```python
from build123d import *

# Parameters (mm, degrees)
SKETCH1_R           = 2.25
SKETCH1_R_2         = 1
SKETCH1_R_3         = 1.65
SKETCH1_W           = 40.6
SKETCH1_H           = 20.8
SKETCH1_W_2         = 23
SKETCH1_H_2         = 12.9
BOSS_EXTRUDE1_DEPTH = 3.175


with BuildPart() as part:
    # Sketch1 → Boss-Extrude1 (new body)
    with BuildSketch(Plane(origin=(0, 0, 0), x_dir=(1, 0, 0), z_dir=(0, 1, 0))):
        with BuildLine():
            Line((-162.38735588, 17.244652891), (-102.38735588, 17.244652891))
            Line((-102.38735588, 17.244652891), (7.61264412, 12.244652891))
            ThreePointArc((7.61264412, 12.244652891), (17.61264412, 2.244652891), (7.61264412, -7.755347109))
            Line((7.61264412, -7.755347109), (-102.38735588, -12.755347109))
            Line((-102.38735588, -12.755347109), (-162.38735588, -12.755347109))
            ThreePointArc((-162.38735588, -12.755347109), (-177.38735588, 2.244652891), (-162.38735588, 17.244652891))
        make_face()
        with Locations(Location((-168.38735588, 7.244652891, 0), (0, 0, 270))):
            Circle(SKETCH1_R, mode=Mode.SUBTRACT)
        with Locations(Location((-168.38735588, -2.755347109, 0), (0, 0, 270))):
            Circle(SKETCH1_R, mode=Mode.SUBTRACT)
        with Locations(Location((-118.78735588, 7.244652891, 0), (0, 0, 270))):
            Circle(SKETCH1_R, mode=Mode.SUBTRACT)
        with Locations(Location((-118.78735588, -2.755347109, 0), (0, 0, 270))):
            Circle(SKETCH1_R, mode=Mode.SUBTRACT)
        with Locations(Location((-15.58735588, 2.244652891, 0), (0, 0, 270))):
            Circle(SKETCH1_R_2, mode=Mode.SUBTRACT)
        with Locations(Location((11.81264412, 2.244652891, 0), (0, 0, 270))):
            Circle(SKETCH1_R_2, mode=Mode.SUBTRACT)
        with Locations(Location((-42.38735588, 2.244652891, 0), (0, 0, 270))):
            Circle(SKETCH1_R_3, mode=Mode.SUBTRACT)
        with Locations((-142.392621679, 2.244652891)):
            Rectangle(SKETCH1_W, SKETCH1_H, mode=Mode.SUBTRACT)
        with Locations((-1.88735588, 2.244652891)):
            Rectangle(SKETCH1_W_2, SKETCH1_H_2, mode=Mode.SUBTRACT)
    extrude(amount=BOSS_EXTRUDE1_DEPTH)


solid = part.part
```
Work out the finished part from the listing and answer in its coordinate system (mm). A direction names the side the tool comes from. Give positions to 0.01 mm unless a question says otherwise; leave off trailing zeros. Loops run counter-clockwise (first coordinate to the right, second up) from the corner with the lowest first, then second, coordinate; pieces in that order, holes last. Notation, with made-up numbers: (-10, -15.5) -> (-3, -15.5) arc R11 cw to (-3, 2.5) -> close; hole circle Ø11 at (-3, -4). An arc over 180 degrees is marked (long way). One line per question, with ' | ' between items. Start each with the question number.
1) Straight lines are drawn through the part: L1, parallel to Z at x = -169, y = 1.45; L2, parallel to X at y = 0.2, z = -8.5; L3, parallel to Z at x = -152.5, y = 1.85. For each, find the intervals that lie inside material, in ascending order.
2) Section B-B, the plane y = 1.4 is taken. State how many separate pieces and enclosed holes the cut face has, then the cut area to 3 significant figures.
3) Section C-C, the plane z = -7 is taken. Determine the outline of the cut face in (x, y) (3 decimals).
4) Determine the mould class of faces 1 (the face through (-133, 2, -17.245)), 2 (the face through (-132, 2, 12.755)), 3 (the face through (-143, 2, 8.155)) for opening direction Z: +Z half, -Z half, draft (parallel to the pull), parting line (faces both ways), or undercut.
5) Section D-D, the plane x = -3 is taken. Determine the outline of the cut face in (y, z) (3 decimals), then the cut area to 3 significant figures.
6) For faces 4 (the face through (-2, 2, -8.695)), 5 (the face through (-177.384, 1.565, -1.915)), determine the directions among +Z, -Z, +X, -X, +Y, -Y from which every point of the face is accessible in a straight line to the end or side of a thin tool.
7) Section A-A, the plane x = -140.5 is taken. Determine the outline of the cut face in (y, z) (3 decimals).
8) Each of these flat-tipped pins is pushed along its axis until it touches: pin 1 (1.8 mm diameter, centred on x = -15.59, z = -2.24, fed in from -Y); pin 2 (1 mm diameter, centred on y = 2, z = -3.5, fed in from +X); pin 3 (1 mm diameter, centred on x = 0.5, y = 1.5, fed in from +Z); pin 4 (1.5 mm diameter, centred on x = -39.5, y = 0.5, fed in from -Z). Where does it stop, or does it pass through?
Resolved:
1) L1: -15.71 to -9.41, -5.08 to 0.59, 4.92 to 11.22 | L2: -176.02 to -170.25, -166.52 to -162.69, -122.09 to -120.65, -116.92 to -13.39, 9.61 to 15.41 | L3: -17.24 to -12.64, 8.16 to 12.76
2) separate pieces: 1 | enclosed holes: 9 | area: 3,840 mm2
3) outline: (-176.614, 0) -> (-170.624, 0) -> (-170.624, 3.175) -> (-176.614, 3.175) -> close; (-166.151, 0) -> (-162.693, 0) -> (-162.693, 3.175) -> (-166.151, 3.175) -> close; (-122.093, 0) -> (-121.024, 0) -> (-121.024, 3.175) -> (-122.093, 3.175) -> close; (-116.551, 0) -> (-13.387, 0) -> (-13.387, 3.175) -> (-116.551, 3.175) -> close; (9.613, 0) -> (16.41, 0) -> (16.41, 3.175) -> (9.613, 3.175) -> close
4) face 1: -Z half | face 2: +Z half | face 3: undercut
5) outline: (0, -12.727) -> (3.175, -12.727) -> (3.175, -8.695) -> (0, -8.695) -> close; (0, 4.205) -> (3.175, 4.205) -> (3.175, 8.238) -> (0, 8.238) -> close | area: 25.6 mm2
6) face 4: +Y, -Y | face 5: -X, +Y, -Y
7) outline: (0, -17.245) -> (3.175, -17.245) -> (3.175, -12.645) -> (0, -12.645) -> close; (0, 8.155) -> (3.175, 8.155) -> (3.175, 12.755) -> (0, 12.755) -> close
8) pin 1: through | pin 2: x = 17.58 | pin 3: z = 8.1 | pin 4: z = -14.42
